Design review of the part built by this model. Coordinates are the model's own, in mm. Face numbers are marked on the shaded views. A direction names the side the tool comes from. Round coordinates to 2 decimals unless told otherwise and drop trailing zeros. Order: outer loops, then holes, each group sorted by start corner. A loop starts at its lowest first (then second) coordinate and runs counter-clockwise, first axis right, second up. Notation, with made-up numbers: (55, 31.5) - (106, 31.5) arc R13 ccw to (106, 35.5) - close; hole circle Ø3 at (-10, 66). An arc over 180 degrees is marked (long way). Answer as a JSON object with one key per item and string values. Group by question number.
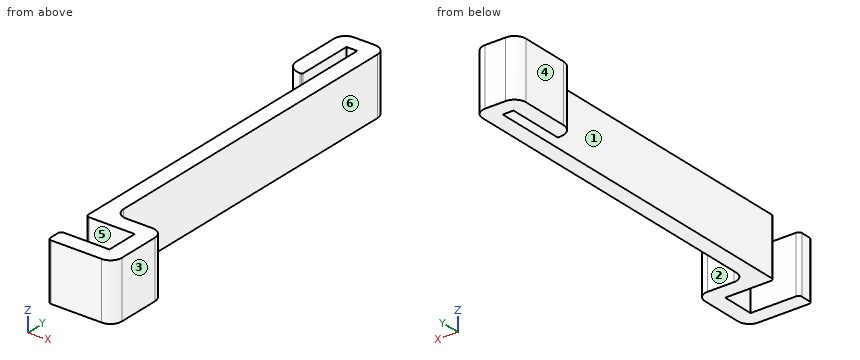
Autodesk Fusion 360 part; units mm, degrees
sketch "Sketch1" plane through (0, 0, 0) normal (0, 0, 1) x (1, 0, 0)
  line L0 (0, 8.5) -> (0, 38)
  line L1 (8.5, 0) -> (9.5, 0)
  line L2 (10, 0.5) -> (10, 35)
  line L3 (10, 35) -> (16.6, 35)
  line L4 (16.6, 35) -> (16.6, -177.5)
  line L5 (18.6, -179.5) -> (26.6, -179.5)
  line L6 (26.6, -162.5) -> (26.6, 38)
  line L7 (19.6, 45) -> (7, 45)
  line L8 (26.6, -179.5) -> (56.6, -179.5)
  line L9 (56.6, -179.5) -> (56.6, -176.5)
  line L10 (49.6, -169.5) -> (33.6, -169.5)
  line L11 (56.6, -179.5) -> (56.6, -202.5)
  line L12 (49.6, -209.5) -> (46.6, -209.5)
  line L13 (46.6, -209.5) -> (46.6, -179.5)
  line L14 (46.6, -209.5) -> (18.6, -209.5)
  line L15 (16.6, -207.5) -> (16.6, -201.5)
  line L16 (18.6, -199.5) -> (46.6, -199.5)
  arc A0 (0, 8.5) -> (8.5, 0) centre (8.5, 8.5) ccw
  arc A1 (9.5, 0) -> (10, 0.5) centre (9.5, 0.5) ccw
  arc A2 (7, 45) -> (0, 38) centre (7, 38) ccw
  arc A3 (26.6, 38) -> (19.6, 45) centre (19.6, 38) ccw
  arc A4 (16.6, -177.5) -> (18.6, -179.5) centre (18.6, -177.5) ccw
  arc A5 (18.6, -199.5) -> (16.6, -201.5) centre (18.6, -201.5) ccw
  arc A6 (16.6, -207.5) -> (18.6, -209.5) centre (18.6, -207.5) ccw
  arc A7 (56.6, -176.5) -> (49.6, -169.5) centre (49.6, -176.5) ccw
  arc A8 (49.6, -209.5) -> (56.6, -202.5) centre (49.6, -202.5) ccw
  arc A9 (26.6, -162.5) -> (33.6, -169.5) centre (33.6, -162.5) ccw
  point P0 (0, 45)
  point P1 (10, 0)
  point P2 (16.6, -179.5)
  point P3 (56.6, -169.5)
  point P4 (56.6, -209.5)
  point P5 (16.6, -209.5)
  point P6 (16.6, -199.5)
  dimension "d1" = 45
  dimension "d2" = 10
  dimension "d3" = 35
  dimension "d4" = 6.6
  dimension "d5" = 10
  dimension "d6" = 214.5
  dimension "d7" = 30
  dimension "d8" = 10
  dimension "d9" = 30
  dimension "d10" = 10
  dimension "d11" = 30
  dimension "d12" = 10
  dimension "d13" = 8.5
  dimension "d14" = 0.5
  dimension "d15" = 7
  dimension "d16" = 7
  dimension "d17" = 2
  dimension "d18" = 2
  dimension "d19" = 2
  dimension "d20" = 7
  dimension "d21" = 7
  dimension "d22" = 7
extrude "Extrude1" add sketch "Sketch1" along normal blind 35
1. Clearance check with flat-ended pins moving along their axes: P1, Ø12, axis at y = -134.5, z = 5, coming from the +X side; P2, Ø17.5, axis at x = 42.5, z = 9, coming from the +Y side; P3, Ø1.1, axis at x = 9, z = 24, coming from the -Y side; P4, Ø2, axis at y = 13, z = 8, coming from the -X side. State where each tip first meets the part, or that it passes through.
2. Take a section at B-B, the plane x = 42.5. Give the boundary of the cut face in (y, z), then the cut area to 3 significant figures.
3. Mouldability with a two-part tool opening along X and no side actions: class the marked faces 1, 2 and 3 as pulls with the +X half, pulls with the -X half, needs draft (parallel to the pull), parting line crosses it, or undercut.
4. Take a section at D-D, the plane y = -58. Give the boundary of the cut face in (x, z), then the cut area to 3 significant figures.
5. To check wall thickness, follow line 1 (X direction, y = 10, z = 14.5); line 2 (Y direction, x = 38.5, z = 4); line 3 (Y direction, x = 20, z = 31.5). State the ranges of each line that lie inside material, in increasing order. Write a range as from..to.
6. Tool access review of the marked faces 4, 5 and 6: name each direction out of +Z, -Z, +X, -X, +Y, -Y from which nothing blocks a thin tool from reaching the whole face with its end or side.
7. Take a section at C-C, the plane z = 13.5. Give the boundary of the cut face in (x, y).
8. Take a section at A-A, the plane y = 6. Give the boundary of the cut face in (x, z).
Response values:
{
 "1": {"P1": "x = 26.6", "P2": "y = -169.5", "P3": "y = 0", "P4": "x = 0"},
 "2": {"outline": "(-209.5, 0) - (-199.5, 0) - (-199.5, 35) - (-209.5, 35) - close; (-179.5, 0) - (-169.5, 0) - (-169.5, 35) - (-179.5, 35) - close", "area": "700 mm2"},
 "3": {"face 1": "undercut", "face 2": "needs draft", "face 3": "pulls with the +X half"},
 "4": {"outline": "(16.6, 0) - (26.6, 0) - (26.6, 35) - (16.6, 35) - close", "area": "350 mm2"},
 "5": {"line 1": "0..10, 16.6..26.6", "line 2": "-209.5..-199.5, -179.5..-169.5", "line 3": "-209.5..-199.5, -179.5..44.99"},
 "6": {"face 4": "+Z, -Z, -X, +Y, -Y", "face 5": "+Z, -Z, -X", "face 6": "+Z, -Z, +X, +Y"},
 "7": {"outline": "(0, 8.5) arc R8.5 ccw to (8.5, 0) - (9.5, 0) arc R0.5 ccw to (10, 0.5) - (10, 35) - (16.6, 35) - (16.6, -177.5) arc R2 ccw to (18.6, -179.5) - (46.6, -179.5) - (46.6, -199.5) - (18.6, -199.5) arc R2 ccw to (16.6, -201.5) - (16.6, -207.5) arc R2 ccw to (18.6, -209.5) - (49.6, -209.5) arc R7 ccw to (56.6, -202.5) - (56.6, -176.5) arc R7 ccw to (49.6, -169.5) - (33.6, -169.5) arc R7 cw to (26.6, -162.5) - (26.6, 38) arc R7 ccw to (19.6, 45) - (7, 45) arc R7 ccw to (0, 38) - close"},
 "8": {"outline": "(0.38, 0) - (10, 0) - (10, 35) - (0.38, 35) - close; (16.6, 0) - (26.6, 0) - (26.6, 35) - (16.6, 35) - close"}
}
